```python
from build123d import *

# Parameters (mm, degrees)
BOSS_EXTRUDE1_DEPTH                 = 19.05
F_1_3_4_CLEARANCE_HOLE1_D           = 45
F_1_3_4_CLEARANCE_HOLE1_DEPTH       = 5
F_1_4_CLEARANCE_HOLE3_D             = 6.6
F_1_4_CLEARANCE_HOLE3_DEPTH         = 19.05
BOSS_EXTRUDE2_DEPTH                 = 19.05
SKETCH21_R                          = 30
CUT_EXTRUDE1_DEPTH                  = 20.05
BOSS_EXTRUDE5_DEPTH                 = 19.05
BOSS_EXTRUDE6_DEPTH                 = 19.05
FILLET2_R                           = 13
SKETCH29_W                          = 12.7
SKETCH29_H                          = 60
BOSS_EXTRUDE7_DEPTH                 = 19.05
BOSS_EXTRUDE8_DEPTH                 = 19.05
FILLET3_R                           = 3.175
F_3_8_0_3750_DOWEL_HOLE1_AT_2_COUNT = 2
F_3_8_0_3750_DOWEL_HOLE1_AT_2_PITCH = 73.92046334
F_4_CLEARANCE_HOLE2_D               = 3.2999934
TAP_DRILL_FOR_1_4_20_TAP1_D         = 5.1054
TAP_DRILL_FOR_1_4_20_TAP1_DEPTH     = 12.7
TAP_DRILL_FOR_1_4_20_TAP1_TIP       = 1.533816902
TAP_DRILL_FOR_1_4_20_TAP2_D         = 5.1054
TAP_DRILL_FOR_1_4_20_TAP2_DEPTH     = 12.7
TAP_DRILL_FOR_1_4_20_TAP2_TIP       = 1.533816902


with BuildPart() as part:
    # Sketch1 → Boss-Extrude1 (new body)
    with BuildSketch(Plane(origin=(0, 0, 0), x_dir=(-1, 0, 0), z_dir=(0, 0, -1))):
        with BuildLine():
            Line((44.45, 0), (44.45, 60))
            Line((44.45, 60), (-44.45, 60))
            Line((-44.45, 60), (-44.45, 0))
            ThreePointArc((-44.45, 0), (0, -44.45), (44.45, 0))
        make_face()
    extrude(amount=-BOSS_EXTRUDE1_DEPTH)

    # 1-3/4 Clearance Hole1
    with Locations(Plane(origin=(0, 0, 0), x_dir=(-1, 0, 0), z_dir=(0, 0, -1))):
        with Locations((-6, 0)):
            Hole(F_1_3_4_CLEARANCE_HOLE1_D / 2, depth=F_1_3_4_CLEARANCE_HOLE1_DEPTH)

    # 1/4 Clearance Hole3
    with Locations(Plane.XY.offset(19.05)):
        with Locations((18.374368671, 12.374368671), (23.499999956, -0.001247108), (18.374368671, -12.374368671), (6, -17.5), (-6.374368671, -12.374368671), (-11.5, 0), (-6.374368671, 12.374368671), (6, 17.5)):
            Hole(F_1_4_CLEARANCE_HOLE3_D / 2, depth=F_1_4_CLEARANCE_HOLE3_DEPTH)

    # Sketch18 → Boss-Extrude2 (add)
    with BuildSketch(Plane(origin=(0, 0, 0), x_dir=(-1, 0, 0), z_dir=(0, 0, -1))):
        with BuildLine():
            Line((-44.45, 0), (-50.45, 0))
            ThreePointArc((-50.45, 0), (-37.430896424, -31.430896424), (-6, -44.45))
            Line((-6, -44.45), (0, -44.45))
            ThreePointArc((0, -44.45), (-31.430896424, -31.430896424), (-44.45, 0))
        make_face()
    extrude(amount=-BOSS_EXTRUDE2_DEPTH)

    # Sketch21 → Cut-Extrude1 (cut, through all)
    with BuildSketch(Plane.XY.offset(19.05)):
        with BuildLine():
            Line((-44.45, 60), (-44.45, 0))
            ThreePointArc((-44.45, 0), (-31.430896424, -31.430896424), (0, -44.45))
            Line((0, -44.45), (6, -44.45))
            ThreePointArc((6, -44.45), (37.430896424, -31.430896424), (50.45, 0))
            Line((50.45, 0), (44.45, 0))
            Line((44.45, 0), (44.45, 60))
            Line((44.45, 60), (-44.45, 60))
        make_face()
        with Locations((5.999999978, -0.000623554)):
            Circle(SKETCH21_R, mode=Mode.SUBTRACT)
    extrude(amount=-CUT_EXTRUDE1_DEPTH, mode=Mode.SUBTRACT)

    # Sketch22 → Boss-Extrude5 (add)
    with BuildSketch(Plane.XY.offset(19.05)):
        with BuildLine():
            Line((44.099999978, -30.000623554), (44.099999978, 29.999376446))
            Line((44.099999978, 29.999376446), (5.999999978, 29.999376446))
            ThreePointArc((5.999999978, 29.999376446), (35.999999978, -0.000623554), (5.999999978, -30.000623554))
            Line((5.999999978, -30.000623554), (44.099999978, -30.000623554))
        make_face()
    boss_extrude5 = extrude(amount=-BOSS_EXTRUDE5_DEPTH)

    # Mirror1: Boss-Extrude5 across plane
    add(boss_extrude5.mirror(Plane(origin=(5.999999978, 0, 0), x_dir=(0, 0, 1), z_dir=(1, 0, 0))))

    # Sketch28 → Boss-Extrude6 (add)
    with BuildSketch(Plane.XY.offset(19.05)):
        with BuildLine():
            Line((-26.798858004, 29.999376446), (38.798858004, 29.999376446))
            ThreePointArc((38.798858004, 29.999376446), (6, 44.448752892), (-26.798858004, 29.999376446))
        make_face()
        with BuildLine():
            ThreePointArc((-26.798858004, -30.000623554), (6, -44.45), (38.798858004, -30.000623554))
            Line((38.798858004, -30.000623554), (-26.798858004, -30.000623554))
        make_face()
    extrude(amount=-BOSS_EXTRUDE6_DEPTH)

    # Fillet2
    fillet2_edges = [part.edges().sort_by_distance(p)[0] for p in [
        (-26.798858004, 29.999376446, 9.525),
        (38.798858004, 29.999376446, 9.525),
        (38.798858004, -30.000623554, 9.525),
        (-26.798858004, -30.000623554, 9.525),
    ]]
    fillet(fillet2_edges, radius=FILLET2_R)

    # Sketch29 → Boss-Extrude7 (add)
    with BuildSketch(Plane.XY):
        with Locations((50.449999978, -0.000623554)):
            Rectangle(SKETCH29_W, SKETCH29_H)
        with Locations((-38.447885426, -0.000623554)):
            Rectangle(SKETCH29_W, SKETCH29_H)
    extrude(amount=BOSS_EXTRUDE7_DEPTH)

    # Sketch40 → Boss-Extrude8 (add)
    with BuildSketch(Plane.XY.offset(19.05)):
        with BuildLine():
            Line((56.799999978, -30.000623554), (44.097885426, -30.000623554))
            ThreePointArc((44.097885426, -30.000623554), (39.487811488, -30.845492198), (35.476953998, -33.27028228))
            ThreePointArc((35.476953998, -33.27028228), (6, -44.45), (-23.476953998, -33.27028228))
            ThreePointArc((-23.476953998, -33.27028228), (-27.487811488, -30.845492198), (-32.097885426, -30.000623554))
            Line((-32.097885426, -30.000623554), (-44.797885426, -30.000623554))
            Line((-44.797885426, -30.000623554), (-44.797885426, -52.835855224))
            Line((-44.797885426, -52.835855224), (-36.33121876, -52.835855224))
            ThreePointArc((-36.33121876, -52.835855224), (6.001057276, -45.572977311), (48.333333311, -52.835855224))
            Line((48.333333311, -52.835855224), (56.799999978, -52.835855224))
            Line((56.799999978, -52.835855224), (56.799999978, -30.000623554))
        make_face()
        with BuildLine():
            Line((-36.33121876, 52.834608116), (-44.797885426, 52.834608116))
            Line((-44.797885426, 52.834608116), (-44.797885426, 29.999376446))
            Line((-44.797885426, 29.999376446), (-32.097885426, 29.999376446))
            ThreePointArc((-32.097885426, 29.999376446), (-27.487811488, 30.84424509), (-23.476953998, 33.269035172))
            ThreePointArc((-23.476953998, 33.269035172), (6, 44.448752892), (35.476953998, 33.269035172))
            ThreePointArc((35.476953998, 33.269035172), (39.487811488, 30.84424509), (44.097885426, 29.999376446))
            Line((44.097885426, 29.999376446), (56.799999978, 29.999376446))
            Line((56.799999978, 29.999376446), (56.799999978, 52.834608116))
            Line((56.799999978, 52.834608116), (48.333333311, 52.834608116))
            ThreePointArc((48.333333311, 52.834608116), (6.001057276, 45.571730203), (-36.33121876, 52.834608116))
        make_face()
    extrude(amount=-BOSS_EXTRUDE8_DEPTH)

    # Fillet3
    fillet3_edges = [part.edges().sort_by_distance(p)[0] for p in [
        (-44.797885426, -52.835855224, 9.525),
        (-36.33121876, -52.835855224, 9.525),
        (48.333333311, -52.835855224, 9.525),
        (56.799999978, -52.835855224, 9.525),
        (56.799999978, 52.834608116, 9.525),
        (48.333333311, 52.834608116, 9.525),
        (-36.33121876, 52.834608116, 9.525),
        (-44.797885426, 52.834608116, 9.525),
    ]]
    fillet(fillet3_edges, radius=FILLET3_R)

    # Sketch49 → 3/8 (0.3750) Dowel Hole1 (revolve, cut)
    with BuildSketch(Plane(origin=(56.799999978, -36.960855224, 9.525), x_dir=(0, 0, -1), z_dir=(0, 1, 0))):
        Polygon((0, 0), (0, 28.261598698), (4.7625, 25.4), (4.7625, 0), align=None)
    f_3_8_0_3750_dowel_hole1 = revolve(axis=Axis((63.149999978, -36.960855224, 9.525), (-1, 0, 0)), mode=Mode.SUBTRACT)

    # 3/8 (0.3750) Dowel Hole1 at 2: 3/8 (0.3750) Dowel Hole1 ×2
    with Locations(*[(0, i * F_3_8_0_3750_DOWEL_HOLE1_AT_2_PITCH, 0) for i in range(1, F_3_8_0_3750_DOWEL_HOLE1_AT_2_COUNT)]):
        add(f_3_8_0_3750_dowel_hole1, mode=Mode.SUBTRACT)

    # Mirror6: 3/8 (0.3750) Dowel Hole1 across plane
    add(f_3_8_0_3750_dowel_hole1.mirror(Plane(origin=(5.999999978, 0, 0), x_dir=(0, 0, 1), z_dir=(1, 0, 0))), mode=Mode.SUBTRACT)

    # Mirror6 copy 1 sketch → Mirror6 copy 1 (revolve, cut)
    with BuildSketch(Plane(origin=(-44.800000022, 36.959608116, 9.525), x_dir=(0, 0, -1), z_dir=(0, 1, 0))):
        Polygon((0, 0), (0, -28.261598698), (4.7625, -25.4), (4.7625, 0), align=None)
    revolve(axis=Axis((-51.150000022, 36.959608116, 9.525), (-1, 0, 0)), mode=Mode.SUBTRACT)

    # #4 Clearance Hole2 (through all)
    with Locations(Plane(origin=(0, 0, 0), x_dir=(-1, 0, 0), z_dir=(0, 0, -1))):
        with Locations((-6, -26.35), (20.35, 0), (-6, 26.35), (-32.35, 0)):
            Hole(F_4_CLEARANCE_HOLE2_D / 2)

    # Tap Drill for 1/4-20 Tap1
    with Locations(Plane.ZY.offset(44.797885426)):
        with Locations((9.525, -0.000623554)):
            Hole(TAP_DRILL_FOR_1_4_20_TAP1_D / 2, depth=TAP_DRILL_FOR_1_4_20_TAP1_DEPTH)
            with Locations((0, 0, -(TAP_DRILL_FOR_1_4_20_TAP1_DEPTH + TAP_DRILL_FOR_1_4_20_TAP1_TIP / 2))):  # 118° drill point
                Cone(0, TAP_DRILL_FOR_1_4_20_TAP1_D / 2, TAP_DRILL_FOR_1_4_20_TAP1_TIP, mode=Mode.SUBTRACT)

    # Tap Drill for 1/4-20 Tap2
    with Locations(Plane(origin=(56.799999978, 0, 0), x_dir=(0, 0, -1), z_dir=(1, 0, 0))):
        with Locations((-9.525, -0.000623554)):
            Hole(TAP_DRILL_FOR_1_4_20_TAP2_D / 2, depth=TAP_DRILL_FOR_1_4_20_TAP2_DEPTH)
            with Locations((0, 0, -(TAP_DRILL_FOR_1_4_20_TAP2_DEPTH + TAP_DRILL_FOR_1_4_20_TAP2_TIP / 2))):  # 118° drill point
                Cone(0, TAP_DRILL_FOR_1_4_20_TAP2_D / 2, TAP_DRILL_FOR_1_4_20_TAP2_TIP, mode=Mode.SUBTRACT)


solid = part.part
```
For this review, take the finished solid that the model builds, in its own axes (mm). A direction names the side the tool comes from. Coordinates: 2 decimals unless noted, no trailing zeros. Loops run counter-clockwise (first coordinate to the right, second up) from the corner with the lowest first, then second, coordinate; pieces in that order, holes last. Notation, with made-up numbers: (21, -8) - (47, -8) arc R13 ccw to (47, 5) - close; hole circle Ø9 at (-17.75, 43.5). An arc over 180 degrees is marked (long way). Use one line per item in the form item = value. Start each with the question number.
1) For faces 1 (the face through (50.361, -1.554, 7.499)), 2 (the face through (5.64, 24.74, 9.66)), 3 (the face through (6, 0, 5)), list the 3-axis set-ups (+Z, -Z, +X, -X, +Y, -Y) from which the entire face can be reached by the end or side of a thin tool; tool diameter is ignored.
2) Take a section at C-C (x = -11.5). State the section outline as (y, z) points, plus the area to 3 significant figures.
3) For pin 1 (7.5 mm diameter, centred on y = 36.96, z = 9.52, fed in from +X); pin 2 (3 mm diameter, centred on x = 13.5, z = 15, fed in from +Y); pin 3 (5.5 mm diameter, centred on y = -36.96, z = 9.52, fed in from -X), all flat-tipped, find the tip position at first contact; note any pin that passes through.
4) Take a section at D-D (z = 17.25). State how many separate pieces and enclosed holes the cut face has, plus the area to 3 significant figures.
5) To check wall thickness, follow probe 1 along Y at (x, z) = (6, 2.15); probe 2 along X at (y, z) = (10.5, 17); probe 3 along Y at (x, z) = (7, 18). State the ranges of each line that lie inside material, in increasing order. Write a range as from..to.
6) Take a section at B-B (y = 26.35). State the section outline as (x, z) points, plus the area to 3 significant figures.
7) Take a section at A-A (x = 6). State the section outline as (y, z) points, plus the area to 3 significant figures.
8) Draft analysis for pull direction X (two halves, no side actions). For faces 4 (the face through (-17.035, -37.781, 9.633)), 5 (the face through (56.8, -1, 14)), 6 (the face through (-18.776, 0.496, 9.658)), state which applies: released by +X, released by -X, zero draft, split by the parting line, or undercut.
From the geometry:
q1.face_1 = +X
q1.face_2 = +Z, -Z
q1.face_3 = -Z
q2.outline = (-46.78, 0) - (-14.14, 0) - (-14.14, 5) - (-3.3, 5) - (-3.3, 19.05) - (-46.78, 19.05) - close; (3.3, 5) - (14.14, 5) - (14.14, 0) - (46.78, 0) - (46.78, 19.05) - (3.3, 19.05) - close
q2.area = 1,550 mm2
q3.pin_1 = 30.79
q3.pin_2 = 45.89
q3.pin_3 = -18.19
q4.separate_pieces = 1
q4.enclosed_holes = 12
q4.area = 9,590 mm2
q5.probe_1 = -45.57..-28, -24.7..-22.5, 22.5..24.7, 28..45.57
q5.probe_2 = -44.8..-9.09, -3.66..15.66, 21.09..56.8
q5.probe_3 = -45.58..-27.66, -25.04..-20.64, -14.36..14.36, 20.64..25.04, 27.66..45.58
q6.outline = (-44.8, 0) - (4.35, 0) - (4.35, 19.05) - (-44.8, 19.05) - close; (7.65, 0) - (56.8, 0) - (56.8, 19.05) - (7.65, 19.05) - close
q6.area = 1,870 mm2
q7.outline = (-45.57, 0) - (-28, 0) - (-28, 19.05) - (-45.57, 19.05) - close; (-24.7, 0) - (-22.5, 0) - (-22.5, 5) - (-20.8, 5) - (-20.8, 19.05) - (-24.7, 19.05) - close; (-14.2, 5) - (14.2, 5) - (14.2, 19.05) - (-14.2, 19.05) - close; (20.8, 5) - (22.5, 5) - (22.5, 0) - (24.7, 0) - (24.7, 19.05) - (20.8, 19.05) - close; (28, 0) - (45.57, 0) - (45.57, 19.05) - (28, 19.05) - close
q7.area = 1,200 mm2
q8.face_4 = released by -X
q8.face_5 = released by +X
q8.face_6 = undercut
